```python
from build123d import *

# Parameters (mm, degrees)
SKETCH1_R           = 39.125
BOSS_EXTRUDE1_DEPTH = 8.75
SKETCH4_R           = 31.083201595
CUT_EXTRUDE1_DEPTH  = 9
BOSS_EXTRUDE3_START = 40
SKETCH5_R           = 35
SKETCH5_R_2         = 31.083201595
BOSS_EXTRUDE3_DEPTH = 40
SKETCH8_R           = 50
BOSS_EXTRUDE4_DEPTH = 5
SKETCH10_R          = 2.75
CUT_EXTRUDE2_DEPTH  = 5
CUT_EXTRUDE3_START  = -5
SKETCH11_R          = 31.083201595
CUT_EXTRUDE3_DEPTH  = 5


with BuildPart() as part:
    # Sketch1 → Boss-Extrude1 (new body)
    with BuildSketch(Plane(origin=(0, 0, 0), x_dir=(1, 0, 0), z_dir=(0, 1, 0))):
        with Locations(Location((0, 0, 0), (0, 0, 270))):
            Circle(SKETCH1_R)
    extrude(amount=BOSS_EXTRUDE1_DEPTH)

    # Sketch4 → Cut-Extrude1 (cut)
    with BuildSketch(Plane.XZ):
        with Locations(Location((0, 0, 0), (0, 0, 270))):
            Circle(SKETCH4_R)
    extrude(amount=-CUT_EXTRUDE1_DEPTH, mode=Mode.SUBTRACT)

    # Sketch5 → Boss-Extrude3 (add)
    with BuildSketch(Plane.XZ.offset(BOSS_EXTRUDE3_START)):
        with Locations(Location((0, 0, 0), (0, 0, 270))):
            Circle(SKETCH5_R)
        with Locations(Location((0, 0, 0), (0, 0, 270))):
            Circle(SKETCH5_R_2, mode=Mode.SUBTRACT)
    extrude(amount=-BOSS_EXTRUDE3_DEPTH)

    # Sketch8 → Boss-Extrude4 (add)
    with BuildSketch(Plane.XZ.offset(40)):
        with Locations(Location((0, 0, 0), (0, 0, 270))):
            Circle(SKETCH8_R)
    extrude(amount=-BOSS_EXTRUDE4_DEPTH)

    # Sketch10 → Cut-Extrude2 (cut)
    with BuildSketch(Plane(origin=(0, -35, 0), x_dir=(1, 0, 0), z_dir=(0, 1, 0))):
        with Locations(Location((0, 42.5, 0), (0, 0, 270))):
            Circle(SKETCH10_R)
        with Locations(Location((42.5, 0, 0), (0, 0, 270))):
            Circle(SKETCH10_R)
        with Locations(Location((0, -42.5, 0), (0, 0, 270))):
            Circle(SKETCH10_R)
        with Locations(Location((-42.5, 0, 0), (0, 0, 270))):
            Circle(SKETCH10_R)
    extrude(amount=-CUT_EXTRUDE2_DEPTH, mode=Mode.SUBTRACT)

    # Sketch11 → Cut-Extrude3 (cut)
    with BuildSketch(Plane(origin=(0, -35, 0), x_dir=(1, 0, 0), z_dir=(0, 1, 0)).offset(CUT_EXTRUDE3_START)):
        with Locations(Location((0, 0, 0), (0, 0, 270))):
            Circle(SKETCH11_R)
    extrude(amount=CUT_EXTRUDE3_DEPTH, mode=Mode.SUBTRACT)


solid = part.part
```
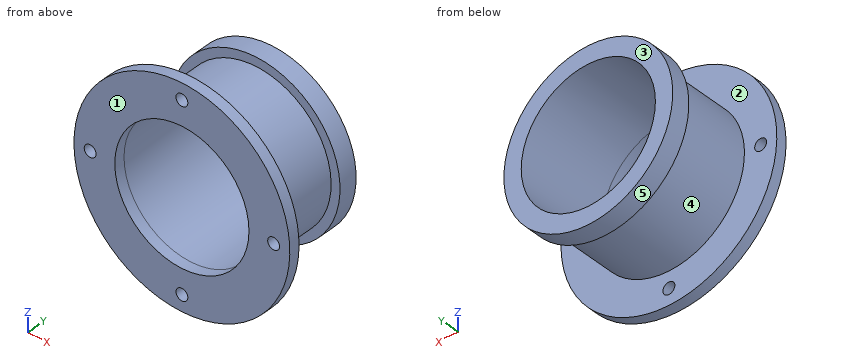
CAD build for the part. Positions are in the model's coordinates, mm. Face numbers are marked on the shaded views. A direction names the side the tool comes from. Round coordinates to 2 decimals unless told otherwise and drop trailing zeros. Write each loop counter-clockwise with the first axis right and the second up, starting at its lowest first coordinate (ties: lowest second). Pieces come first, ordered by that corner, then holes. Notation, with made-up numbers: (79, -38.75) -> (119, -38.75) arc R27 cw to (119, -20.75) -> close; hole circle Ø2 at (40.25, -12.75). An arc over 180 degrees is marked (long way). Answer in a Markdown table with one row per item. Add a question column.
Item 1: Drop flat-ended pins along their axis: pin 1 Ø5 at (x, z) = (0, 42.5) entering from +Y; pin 2 Ø6 at (x, y) = (24, -27.5) entering from -Z; pin 3 Ø12 at (x, y) = (-37, -4.5) entering from +Z; pin 4 Ø10 at (x, y) = (5.5, -13.5) entering from -Z. Give the stop position or say it passes through.
Item 2: Saw through at B-B, the plane z = 42.5. Write the cut outline in (x, y), then the cut area to 3 significant figures.
Item 3: Saw through at D-D, the plane y = 4.5. Write the cut outline in (x, z) (3 decimals), then the cut area to 3 significant figures.
Item 4: Which spindle directions (+Z, -Z, +X, -X, +Y, -Y) get a long thin tool onto all of the face, cutting with end or side? Do the marked faces 4 and 5. Say none if no direction does.
Item 5: Drill centre lines: line 1 (X direction, y = -38.5, z = 0); line 2 (Y direction, x = 34.5, z = -9.5); line 3 (Y direction, x = -12, z = 41.5). Where is each one in solid material? Low to high. Write a range as from..to.
Item 6: Mould opens along Y. For the marked faces 1, 2 and 3 say: pulls with the +Y half, pulls with the -Y half, needs draft (parallel to the pull), parting line crosses it, or undercut.
Item 7: Saw through at C-C, the plane x = -42.5. Write the cut outline in (y, z), then the cut area to 3 significant figures.
Item 8: Saw through at A-A, the plane x = 0. Write the cut outline in (y, z) (3 decimals), then the cut area to 3 significant figures.
Findings below:
| question | item | result |
|---|---|---|
| 1 | pin 1 | passes through |
| 1 | pin 2 | stops at z = -28 |
| 1 | pin 3 | stops at z = 20.97 |
| 1 | pin 4 | stops at z = -35 |
| 2 | outline | (-26.34, -40) -> (-2.75, -40) -> (-2.75, -35) -> (-26.34, -35) -> close; (2.75, -40) -> (26.34, -40) -> (26.34, -35) -> (2.75, -35) -> close |
| 2 | area | 236 mm^2 |
| 3 | outline | circle Ø78.25 at (0, 0); hole circle Ø62.166 at (0, 0) |
| 3 | area | 1,770 mm^2 |
| 4 | face 4 | none |
| 4 | face 5 | +Y |
| 5 | line 1 | x = -50..-45.25, -39.75..-31.08, 31.08..39.75, 45.25..50 |
| 5 | line 2 | y = -40..-35, 0..8.75 |
| 5 | line 3 | y = -40..-35 |
| 6 | face 1 | pulls with the -Y half |
| 6 | face 2 | undercut |
| 6 | face 3 | pulls with the +Y half |
| 7 | outline | (-40, -26.34) -> (-35, -26.34) -> (-35, -2.75) -> (-40, -2.75) -> close; (-40, 2.75) -> (-35, 2.75) -> (-35, 26.34) -> (-40, 26.34) -> close |
| 7 | area | 236 mm^2 |
| 8 | outline | (-40, -50) -> (-35, -50) -> (-35, -45.25) -> (-40, -45.25) -> close; (-40, -39.75) -> (-35, -39.75) -> (-35, -35) -> (0, -35) -> (0, -39.125) -> (8.75, -39.125) -> (8.75, -31.083) -> (-40, -31.083) -> close; (-40, 31.083) -> (8.75, 31.083) -> (8.75, 39.125) -> (0, 39.125) -> (0, 35) -> (-35, 35) -> (-35, 39.75) -> (-40, 39.75) -> close; (-40, 45.25) -> (-35, 45.25) -> (-35, 50) -> (-40, 50) -> close |
| 8 | area | 549 mm^2 |
